For this review, take the finished solid that the model builds, in its own axes (mm). A direction names the side the tool comes from. Round coordinates to 2 decimals unless told otherwise and drop trailing zeros. Order: outer loops, then holes, each group sorted by start corner. A loop starts at its lowest first (then second) coordinate and runs counter-clockwise, first axis right, second up. Notation, with made-up numbers: M 72,64 L 121,64 A30 ccw 121,100 Z; hole C -26.75,51 d4. An arc over 180 degrees is marked long. Answer as a JSON object with one key per item and string values.
from build123d import *

# Parameters (mm, degrees)
F1_DEPTH = 8
F2_W     = 4
F2_H     = 2
F3_DEPTH = 4.2
F4_W     = 4
F4_H     = 2
F5_DEPTH = 4.1
F6_R     = 1.5
F7_DEPTH = 5


with BuildPart() as f1:
    # F0 (on Top) → F1 (new body)
    with BuildSketch(Plane.XY):
        Polygon((-28, 7.5), (-28, -13.5), (-24, -13.5), (-24, 5.5), (-20, 9.5), (20, 9.5), (24, 5.5), (24, -13.5), (28, -13.5), (28, 7.50455), (22, 13.5), (-22, 13.5), align=None)
    extrude(amount=F1_DEPTH)

    # F2 (on face) → F3 (cut)
    with BuildSketch(Plane.YZ.offset(28)):
        with Locations((-11.5, 7)):
            Rectangle(F2_W, F2_H)
        with Locations((-11.5, 1)):
            Rectangle(F2_W, F2_H)
    extrude(amount=-F3_DEPTH, mode=Mode.SUBTRACT)

    # F4 (on face) → F5 (cut)
    with BuildSketch(Plane(origin=(-28, 0, 0), x_dir=(0, -1, 0), z_dir=(-1, 0, 0))):
        with Locations((11.5, 1)):
            Rectangle(F4_W, F4_H)
        with Locations((11.5, 7)):
            Rectangle(F4_W, F4_H)
    extrude(amount=-F5_DEPTH, mode=Mode.SUBTRACT)

    # F6 (on face) → F7 (cut)
    with BuildSketch(Plane(origin=(0, 13.5, 0), x_dir=(-1, 0, 0), z_dir=(0, 1, 0))):
        with Locations((0, 4)):
            Circle(F6_R)
    extrude(amount=-F7_DEPTH, mode=Mode.SUBTRACT)


solid = f1.part
1) Add section D-D on z = 4. State the section outline as (x, y) points.
Geometry check:
{"outline": "M -28,-13.5 L -24,-13.5 L -24,5.5 L -20,9.5 L -1.5,9.5 L -1.5,13.5 L -22,13.5 L -28,7.5 Z; M 1.5,9.5 L 20,9.5 L 24,5.5 L 24,-13.5 L 28,-13.5 L 28,7.5 L 22,13.5 L 1.5,13.5 Z"}
2) Machinability: for faces 4 (the flat face through (25, 10.5, 3.9)), 5 (the flat face through (26, -9.5, 7)), 6 (the flat face through (-26, -11, 2)), 7 (the flat face through (22, 7.5, 3.9)), which of the approach directions +Z, -Z, +X, -X, +Y, -Y give a long, thin tool a straight path to every point of the face, cutting with its end or side? Answer none if there is none.
Geometry check:
{"face 4": "+Z, -Z, +X, +Y", "face 5": "+Z, +X, -X, -Y", "face 6": "-Z, +X, -X, -Y", "face 7": "+Z, -Z, -Y"}
3) Add section A-A on x = 0. State the section outline as (y, z) points, and give its area (3 significant figures).
Geometry check:
{"outline": "M 9.5,0 L 13.5,0 L 13.5,2.5 L 9.5,2.5 Z; M 9.5,5.5 L 13.5,5.5 L 13.5,8 L 9.5,8 Z", "area": "20.0 mm²"}
4) Insertion check: P1, Ø3, axis at x = -27, y = -11.5, coming from the +Z side; P2, Ø1, axis at x = 25, z = 0.5, coming from the -Y side; P3, Ø8, axis at x = 17, y = -4, coming from the +Z side (3 decimals). Each pin has a flat end and moves straight along its axis. Give the tip position at first contact, or say it passes through.
Geometry check:
{"P1": "stops at z = 6", "P2": "stops at y = -9.5", "P3": "passes through"}
5) Mouldability with a two-part tool opening along X and no side actions: class faces 1 (the cylindrical face through (-0.806, 11.528, 5.265)), 2 (the flat face through (0, 10, 8)), 3 (the flat face through (-28, -3, 4)) as +X half, -X half, draft (parallel to the pull), parting line (faces both ways), or undercut.
Geometry check:
{"face 1": "undercut", "face 2": "draft", "face 3": "-X half"}
6) Add section B-B on z = 7.25. State the section outline as (x, y) points, and give its area (3 significant figures).
Geometry check:
{"outline": "M -28,-9.5 L -24,-9.5 L -24,5.5 L -20,9.5 L 20,9.5 L 24,5.5 L 24,-9.5 L 28,-9.5 L 28,7.5 L 22,13.5 L -22,13.5 L -28,7.5 Z", "area": "356 mm²"}
7) Add section C-C on y = -4.75. State the section outline as (x, z) points, and give its area (3 significant figures).
Geometry check:
{"outline": "M -28,0 L -24,0 L -24,8 L -28,8 Z; M 24,0 L 28,0 L 28,8 L 24,8 Z", "area": "64.0 mm²"}
8) For L1, parallel to X at y = -10.75, z = 4; L2, parallel to Z at x = 0, y = 10.5; L3, parallel to Y at x = 21.5, z = 5, list the stretches that pass through material, from the lowest coordinate up.
Geometry check:
{"L1": "x = -28 to -24, 24 to 28", "L2": "z = 0 to 2.5, 5.5 to 8", "L3": "y = 8 to 13.5"}
